Geometry check sheet. Reference: the model listing, model coordinates, mm. A direction names the side the tool comes from. Coordinates: 2 decimals unless noted, no trailing zeros. Loops run counter-clockwise (first coordinate to the right, second up) from the corner with the lowest first, then second, coordinate; pieces in that order, holes last. Notation, with made-up numbers: (-28.5, -20.75) -> (-17.5, -20.75) arc R36 cw to (-17.5, 14.25) -> close; hole circle Ø6 at (-32, 59.5). An arc over 180 degrees is marked (long way). Answer as a JSON object with one key per item and string values.
from build123d import *

# Parameters (mm, degrees)
SKETCH1_W           = 170
SKETCH1_H           = 145
BOSS_EXTRUDE1_DEPTH = 5
SKETCH2_W           = 150
SKETCH2_H           = 125
SKETCH2_W_2         = 145
SKETCH2_H_2         = 120
CUT_EXTRUDE1_DEPTH  = 2.5
SKETCH4_W           = 67.9
SKETCH4_H           = 98.9
SKETCH4_W_2         = 62.9
SKETCH4_H_2         = 93.9
BOSS_EXTRUDE2_DEPTH = 15


with BuildPart() as part:
    # Sketch1 → Boss-Extrude1 (new body)
    with BuildSketch(Plane(origin=(0, 0, 0), x_dir=(1, 0, 0), z_dir=(0, 1, 0))):
        Rectangle(SKETCH1_W, SKETCH1_H)
    extrude(amount=BOSS_EXTRUDE1_DEPTH)

    # Sketch2 → Cut-Extrude1 (cut)
    with BuildSketch(Plane(origin=(0, 5, 0), x_dir=(1, 0, 0), z_dir=(0, 1, 0))):
        Rectangle(SKETCH2_W, SKETCH2_H)
        Rectangle(SKETCH2_W_2, SKETCH2_H_2, mode=Mode.SUBTRACT)
    extrude(amount=-CUT_EXTRUDE1_DEPTH, mode=Mode.SUBTRACT)

    # Sketch4 → Boss-Extrude2 (add)
    with BuildSketch(Plane(origin=(0, 5, 0), x_dir=(1, 0, 0), z_dir=(0, 1, 0))):
        with Locations((0, -10.55)):
            Rectangle(SKETCH4_W, SKETCH4_H)
        with Locations((0, -10.55)):
            Rectangle(SKETCH4_W_2, SKETCH4_H_2, mode=Mode.SUBTRACT)
    extrude(amount=BOSS_EXTRUDE2_DEPTH)


solid = part.part
1. Depth check by flat-ended pin: P1, Ø1.5, axis at y = 10.5, z = 40, coming from the -X side; P2, Ø5, axis at y = 9.5, z = -26, coming from the +X side; P3, Ø10, axis at x = -39, z = 43, coming from the -Y side; P4, Ø4.5, axis at x = -5.5, y = 11, coming from the -Z side. Enter the tip coordinate at first touch or a pass-through.
Evaluation:
{"P1": "stops at x = -33.95", "P2": "stops at x = 33.95", "P3": "stops at y = 0", "P4": "stops at z = -38.9"}
2. Section check A-A, the plane z = -31.5. Record the boundary of the cut face in (x, y).
Evaluation:
{"outline": "(-85, 0) -> (85, 0) -> (85, 5) -> (75, 5) -> (75, 2.5) -> (72.5, 2.5) -> (72.5, 5) -> (33.95, 5) -> (33.95, 20) -> (31.45, 20) -> (31.45, 5) -> (-31.45, 5) -> (-31.45, 20) -> (-33.95, 20) -> (-33.95, 5) -> (-72.5, 5) -> (-72.5, 2.5) -> (-75, 2.5) -> (-75, 5) -> (-85, 5) -> close"}
3. Section check D-D, the plane z = -55. Record the boundary of the cut face in (x, y).
Evaluation:
{"outline": "(-85, 0) -> (85, 0) -> (85, 5) -> (75, 5) -> (75, 2.5) -> (72.5, 2.5) -> (72.5, 5) -> (-72.5, 5) -> (-72.5, 2.5) -> (-75, 2.5) -> (-75, 5) -> (-85, 5) -> close"}
4. Section check C-C, the plane x = -16. Record the boundary of the cut face in (y, z), then the cut area to 4 significant figures.
Evaluation:
{"outline": "(0, -72.5) -> (5, -72.5) -> (5, -62.5) -> (2.5, -62.5) -> (2.5, -60) -> (5, -60) -> (5, -38.9) -> (20, -38.9) -> (20, -36.4) -> (5, -36.4) -> (5, 57.5) -> (20, 57.5) -> (20, 60) -> (2.5, 60) -> (2.5, 62.5) -> (5, 62.5) -> (5, 72.5) -> (0, 72.5) -> close", "area": "787.5 mm^2"}
5. Tool access check on faces 1 (the face through (31.45, 12, 11)), 2 (the face through (0, 12, -38.9)), 3 (the face through (-1, 2, 72.5)). Record the directions out of +Z, -Z, +X, -X, +Y, -Y that give a thin tool (end or side, any length) a straight path to the whole face; none if there is none.
Evaluation:
{"face 1": "+Y", "face 2": "-Z, +X, -X, +Y", "face 3": "+Z, +X, -X, +Y, -Y"}
6. Thickness scan on probe 1 along Z at (x, y) = (-21.5, 3.75); probe 2 along X at (y, z) = (3.75, -2.5); probe 3 along X at (y, z) = (11.75, -16). Record the ranges inside material, lowest first. Write a range as from..to.
Evaluation:
{"probe 1": "z = -72.5..-62.5, -60..60, 62.5..72.5", "probe 2": "x = -85..-75, -72.5..72.5, 75..85", "probe 3": "x = -33.95..-31.45, 31.45..33.95"}
7. Mould release check, pull along X, two halves, no side actions. Record for faces 4 (the face through (33.95, 12, 11)), 5 (the face through (-33.95, 12, 11)), 6 (the face through (-1, 5, -41)), 7 (the face through (0, 5, 10)): released by +X, released by -X, zero draft, split by the parting line, or undercut.
Evaluation:
{"face 4": "released by +X", "face 5": "released by -X", "face 6": "zero draft", "face 7": "undercut"}
8. Section check B-B, the plane y = 18. Record the boundary of the cut face in (x, z).
Evaluation:
{"outline": "(-33.95, -38.9) -> (33.95, -38.9) -> (33.95, 60) -> (-33.95, 60) -> close; hole (-31.45, -36.4) -> (31.45, -36.4) -> (31.45, 57.5) -> (-31.45, 57.5) -> close"}
